Geometry check sheet. Reference: drawing and pictorial views, mm from the part's lowest x, y, z. A direction names the side the tool comes from. Give positions to 0.01 mm unless a question says otherwise; leave off trailing zeros. Write each loop counter-clockwise with the first axis right and the second up, starting at its lowest first coordinate (ties: lowest second). Pieces come first, ordered by that corner, then holes. Notation, with made-up numbers: M -6.75,-30 L 48.25,-30 A30 cw 48.25,5 Z; hole C -23,-28.5 d7. An arc over 180 degrees is marked long. One line per item, written item: value. Start each with the question number.
1. Tool access check on the marked faces 4, 5 and 6. Record the directions out of +Z, -Z, +X, -X, +Y, -Y that give a thin tool (end or side, any length) a straight path to the whole face; none if there is none.
2. Cross-section at C-C on y = 3. Record the cut outline in (x, z) (1 decimal).
3. Cross-section at B-B on x = 6.35. Record the cut outline in (y, z).
4. Scan lines: line 1 (X direction, y = 6.25, z = 7) (1 decimal); line 2 (X direction, y = 6.25, z = 2.5) (1 decimal); line 3 (Y direction, x = 6.35, z = 4.25). Record each from-to range of solid material in increasing order.
5. Gauge pin test, flat ends, axial feed: pin 1 (1 mm diameter, centred on y = 2.5, z = 2.5, fed in from -X) (1 decimal); pin 2 (0.8 mm diameter, centred on y = 7.5, z = 2, fed in from +X); pin 3 (2 mm diameter, centred on y = 6, z = 6, fed in from -X). Record the tip position at first contact, or that the pin passes through.
6. Release check for a two-part mould opening along X. For the marked faces 1, 2 and 3 record: pulls with the +X half, pulls with the -X half, needs draft (parallel to the pull), parting line crosses it, or undercut.
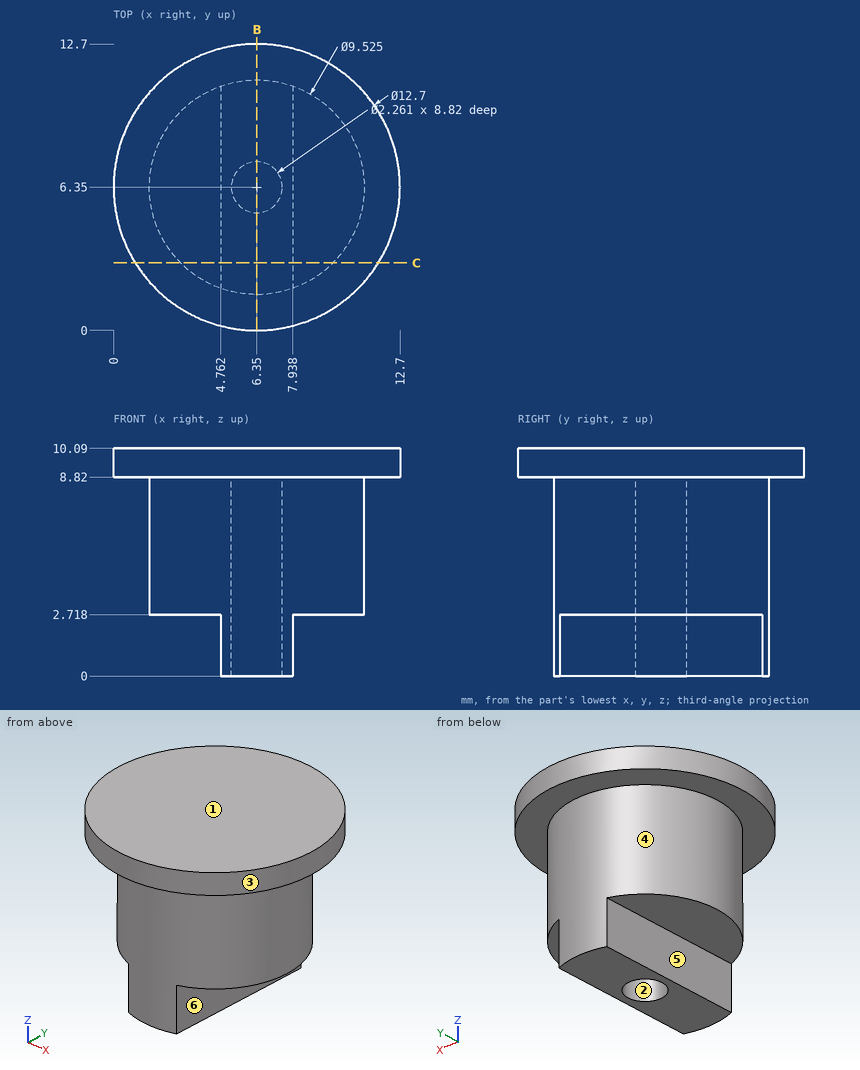
Report:
1. face 4: -Z
1. face 5: -Z, -X, +Y, -Y
1. face 6: -Z, +X, +Y, -Y
2. outline: M 1,8.8 L 3,8.8 L 3,2.7 L 4.8,2.7 L 4.8,0 L 7.9,0 L 7.9,2.7 L 9.7,2.7 L 9.7,8.8 L 11.7,8.8 L 11.7,10.1 L 1,10.1 Z
3. outline: M 0,8.82 L 1.59,8.82 L 1.59,0 L 5.22,0 L 5.22,8.82 L 7.48,8.82 L 7.48,0 L 11.11,0 L 11.11,8.82 L 12.7,8.82 L 12.7,10.09 L 0,10.09 Z
4. line 1: x = 1.6 to 5.2, 7.5 to 11.1
4. line 2: x = 4.8 to 5.2, 7.5 to 7.9
4. line 3: y = 1.59 to 5.22, 7.48 to 11.11
5. pin 1: stops at x = 3
5. pin 2: stops at x = 7.94
5. pin 3: stops at x = 1.59
6. face 1: needs draft
6. face 2: undercut
6. face 3: parting line crosses it
